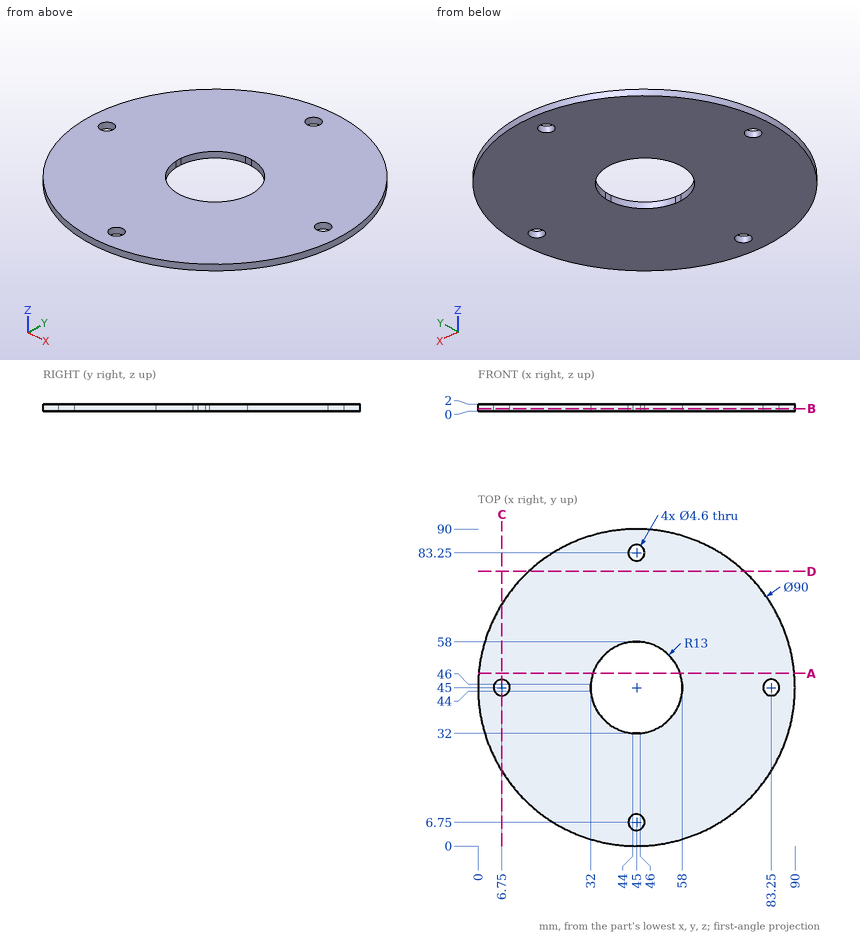
Job drawing, mm, ordinate dimensions from the low corner. One solid piece. Give positions to 0.01 mm unless a question says otherwise; leave off trailing zeros. Loops run counter-clockwise (first coordinate to the right, second up) from the corner with the lowest first, then second, coordinate; pieces in that order, holes last.
Item 1: Drill centre lines: line 1 (Y direction, x = 45, z = 1.1); line 2 (X direction, y = 56, z = 0.7); line 3 (X direction, y = 52, z = 0.1). Where is each one in solid material? Low to high.
Answers follow:
line 1: y = 0 to 4.45, 9.05 to 32, 58 to 80.95, 85.55 to 90
line 2: x = 1.37 to 38.07, 51.93 to 88.63
line 3: x = 0.55 to 34.05, 55.95 to 89.45
Item 2: Slice it at B-B, the plane z = 0.7. Give the number of separate pieces and of enclosed holes in the cut face, and give its area (3 significant figures).
Answers follow:
separate pieces: 1
enclosed holes: 5
area: 5,760 mm2
Item 3: Flat gauge pin, fed straight in: pin 1 (1 mm diameter, centred on x = 45.5, z = 1.5, fed in from -Y). Where does the tip first touch, or does it go through?
Answers follow:
pin 1: stops at y = 0
Item 4: Slice it at C-C, the plane x = 6.75. List the corners of the cut face in (y, z), and give its area (3 significant figures).
Answers follow:
outline: (21.29, 0) - (42.7, 0) - (42.7, 2) - (21.29, 2) - close; (47.3, 0) - (68.71, 0) - (68.71, 2) - (47.3, 2) - close
area: 85.6 mm2
Item 5: Slice it at D-D, the plane y = 78. List the corners of the cut face in (x, z).
Answers follow:
outline: (14.41, 0) - (75.59, 0) - (75.59, 2) - (14.41, 2) - close
Item 6: Slice it at A-A, the plane y = 49. List the corners of the cut face in (x, z).
Answers follow:
outline: (0.18, 0) - (32.63, 0) - (32.63, 2) - (0.18, 2) - close; (57.37, 0) - (89.82, 0) - (89.82, 2) - (57.37, 2) - close
